The figure shows three views and two pictorial views of one solid part (mm, origin at its lowest corner). Answer the questions. Coordinates: 2 decimals unless noted, no trailing zeros. Write each loop counter-clockwise with the first axis right and the second up, starting at its lowest first coordinate (ties: lowest second). Pieces come first, ordered by that corner, then holes. Notation, with made-up numbers: M -27.5,16 L 6.5,16 A21 ccw 6.5,39 Z; hole C 72,70.5 d7. An arc over 180 degrees is marked long. Use a Markdown table: item, result. Add a question column.
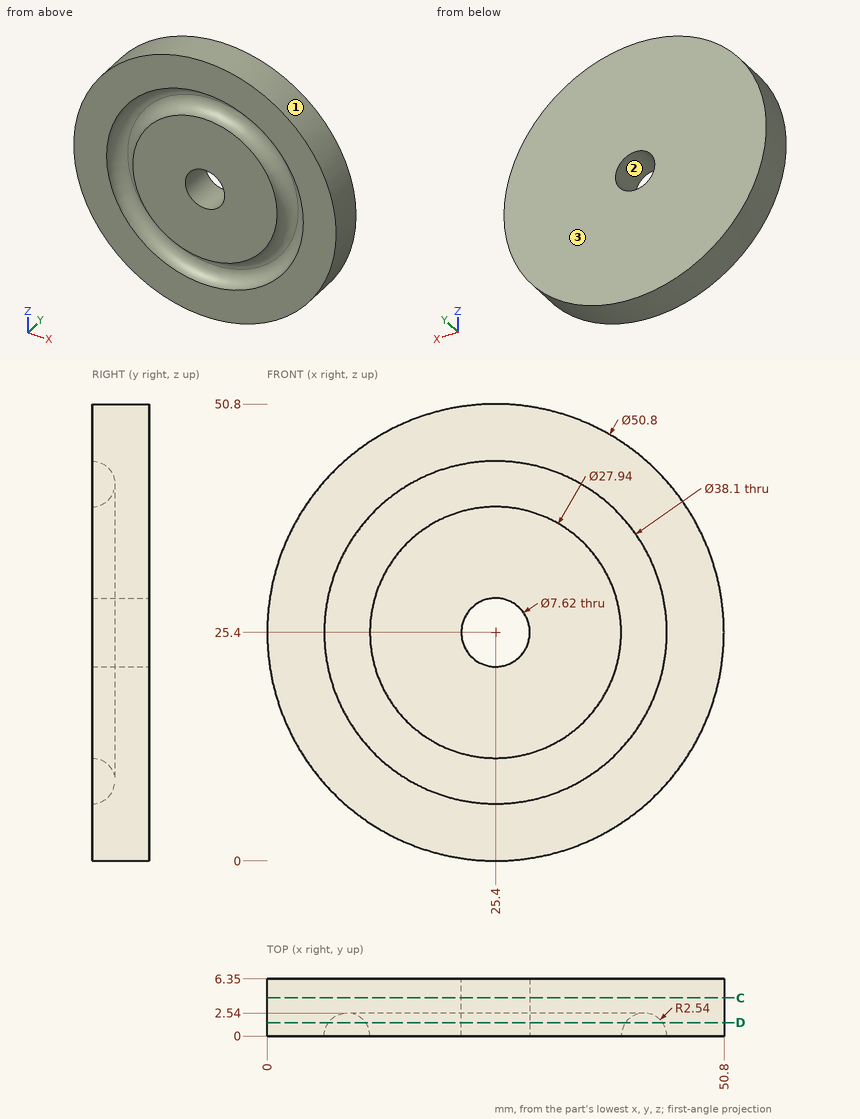
Item 1: Consider probe 1 along Z at (x, y) = (25.4, 0.05); probe 2 along Z at (x, y) = (25.4, 1.75); probe 3 along X at (y, z) = (1, 20). Determine where each line is inside the solid, lowest interval first.
Item 2: Each of these flat-tipped pins is pushed along its axis until it touches: pin 1 (3 mm diameter, centred on y = 3.5, z = 18.5, fed in from -X); pin 2 (6 mm diameter, centred on x = 25.4, z = 25.4, fed in from -Y); pin 3 (2 mm diameter, centred on y = 1.5, z = 20, fed in from -X). Where does it stop, or does it pass through?
Item 3: Find section D-D on y = 1.5. Give the vertices of the cut face in (x, z).
Item 4: Determine the mould class of the marked faces 1, 2 and 3 for opening direction X: pulls with the +X half, pulls with the -X half, needs draft (parallel to the pull), parting line crosses it, or undercut.
Item 5: Find section C-C on y = 4.25. Give the vertices of the cut face in (x, z).
Geometry says:
| question | item | result |
|---|---|---|
| 1 | probe 1 | z = 0 to 6.35, 11.43 to 21.59, 29.21 to 39.37, 44.45 to 50.8 |
| 1 | probe 2 | z = 0 to 7.05, 10.73 to 21.59, 29.21 to 40.07, 43.75 to 50.8 |
| 1 | probe 3 | x = 0.58 to 7.35, 12.29 to 38.51, 43.45 to 50.22 |
| 2 | pin 1 | stops at x = 0.58 |
| 2 | pin 2 | passes through |
| 2 | pin 3 | stops at x = 0.38 |
| 3 | outline | C 25.4,25.4 d50.8; C 25.4,25.4 d28.92; hole C 25.4,25.4 d37.12; hole C 25.4,25.4 d7.62 |
| 4 | face 1 | parting line crosses it |
| 4 | face 2 | undercut |
| 4 | face 3 | needs draft |
| 5 | outline | C 25.4,25.4 d50.8; hole C 25.4,25.4 d7.62 |
